Answer from the drawing. Dimensions are ordinates in mm from the lowest x, y and z of the part. A direction names the side the tool comes from. Coordinates: 2 decimals unless noted, no trailing zeros. Order: outer loops, then holes, each group sorted by start corner. A loop starts at its lowest first (then second) coordinate and runs counter-clockwise, first axis right, second up. Notation, with made-up numbers: M 59,-24.75 L 94,-24.75 A15 cw 94,-7.75 Z; hole C 25,87.25 d6. An arc over 180 degrees is marked long. One line per question, with ' | ' between items. Start each with the question number.
1) Consider probe 1 along X at (y, z) = (7, 49); probe 2 along Z at (x, y) = (8, 7); probe 3 along Z at (x, y) = (57, 78.65). Determine where each line is inside the solid, lowest interval first.
2) Find section C-C, the plane z = 39. Write down the section's boundary in (x, y).
3) Find section B-B, the plane x = 8. Write down the section's boundary in (y, z).
4) Find section D-D, the plane y = 54.5. Write down the section's boundary in (x, z), plus the area to 3 significant figures.
5) A tool of negligible diameter and unlimited length cuts with its end or side. For the marked faces 4, 5 and 6, from which of +Z, -Z, +X, -X, +Y, -Y can it reach the whole face along a straight path? Write none if from no direction.
6) Given P1, Ø9, axis at x = 106, z = 49.1, coming from the +Y side; P2, Ø1, axis at y = 48, z = 29.5, coming from the +X side; P3, Ø16.5, axis at x = 9.5, z = 23, coming from the +Y side, each flat-ended and moving along its own axis, determine where each tip first touches the part or whether it passes through.
7) Find section A-A, the plane z = 8. Write down the section's boundary in (x, y), plus the area to 4 significant figures.
8) The mould has two halves that part along Z. Classify the marked faces 1, 2 and 3: +Z half, -Z half, draft (parallel to the pull), parting line (faces both ways), or undercut.
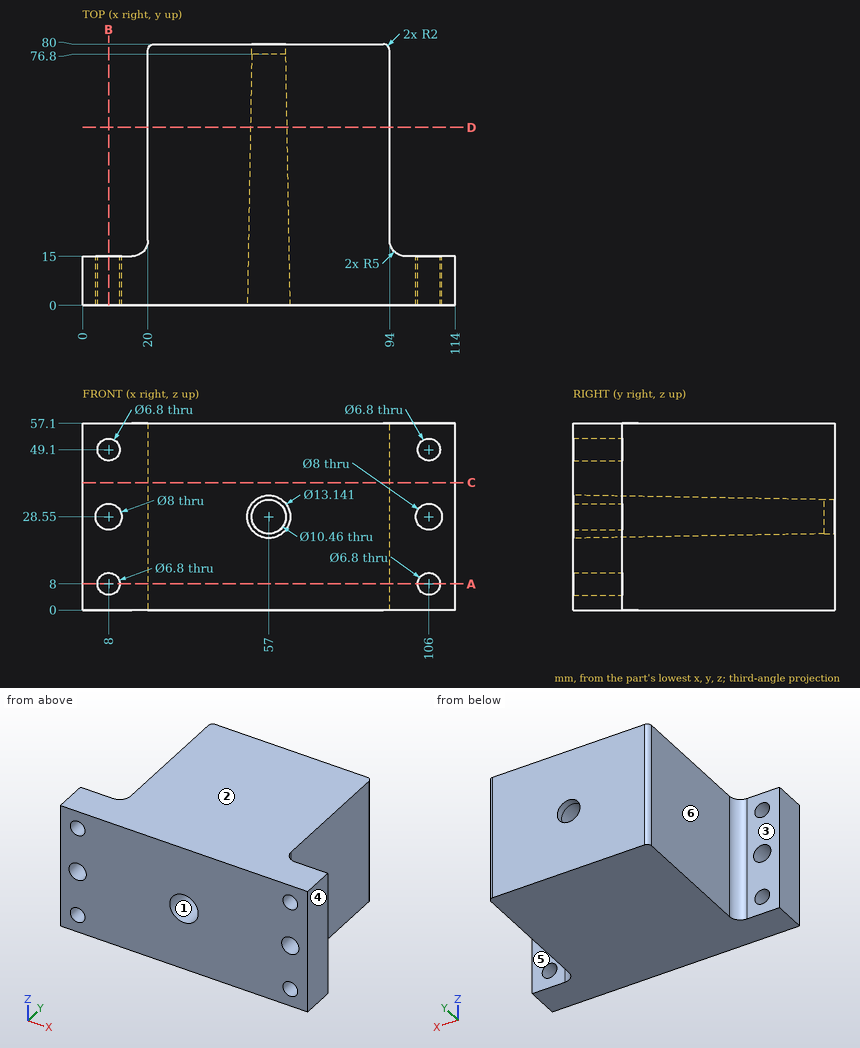
Report:
1) probe 1: x = 0 to 4.6, 11.4 to 102.6, 109.4 to 114 | probe 2: z = 0 to 4.6, 11.4 to 24.55, 32.55 to 45.7, 52.5 to 57.1 | probe 3: z = 0 to 23.32, 33.78 to 57.1
2) outline: M 0,0 L 114,0 L 114,15 L 99,15 A5 cw 94,20 L 94,78 A2 ccw 92,80 L 22,80 A2 ccw 20,78 L 20,20 A5 cw 15,15 L 0,15 Z
3) outline: M 0,0 L 15,0 L 15,4.6 L 0,4.6 Z; M 0,11.4 L 15,11.4 L 15,24.55 L 0,24.55 Z; M 0,32.55 L 15,32.55 L 15,45.7 L 0,45.7 Z; M 0,52.5 L 15,52.5 L 15,57.1 L 0,57.1 Z
4) outline: M 20,0 L 94,0 L 94,57.1 L 20,57.1 Z; hole C 57,28.55 d11.24 | area: 4,130 mm^2
5) face 4: +Z, -Z, +X, +Y, -Y | face 5: +Z, -Z, +X, +Y | face 6: +Z, -Z, -X, +Y
6) P1: stops at y = 15 | P2: stops at x = 94 | P3: stops at y = 15.82
7) outline: M 0,0 L 4.6,0 L 4.6,15 L 0,15 Z; M 11.4,0 L 102.6,0 L 102.6,15 L 99,15 A5 cw 94,20 L 94,78 A2 ccw 92,80 L 22,80 A2 ccw 20,78 L 20,20 A5 cw 15,15 L 11.4,15 Z; M 109.4,0 L 114,0 L 114,15 L 109.4,15 Z | area: 6,325 mm^2
8) face 1: undercut | face 2: +Z half | face 3: draft
